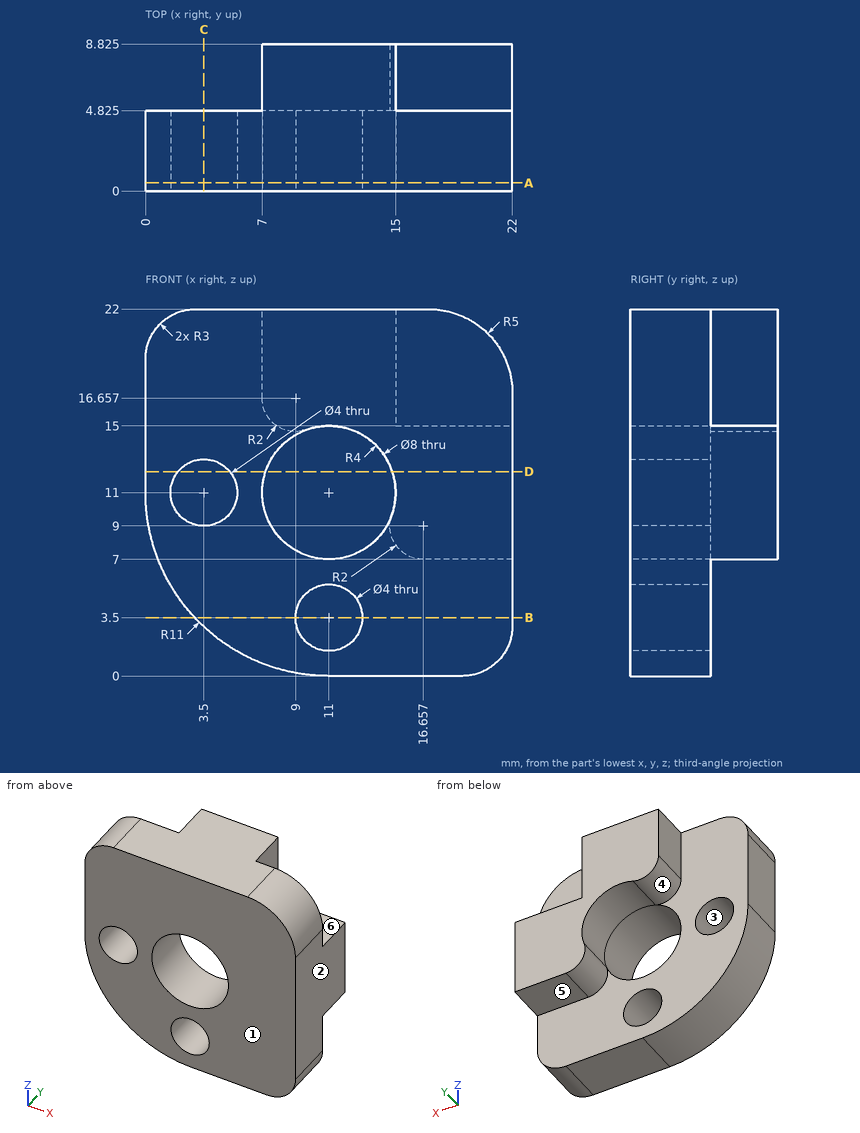
Geometry: see drawing. Coordinates: mm, zero at the bounding-box minimum. A direction names the side the tool comes from. Give positions to 0.01 mm unless a question says otherwise; leave off trailing zeros. Loops run counter-clockwise (first coordinate to the right, second up) from the corner with the lowest first, then second, coordinate; pieces in that order, holes last. Notation, with made-up numbers: M 22,27.5 L 29,27.5 A28 cw 29,61.5 Z; hole C -36.5,37 d8. An arc over 180 degrees is marked long. Use one line per item in the form item = value.
1. Pull-direction query (X, two-part tool) for the marked faces 1, 2 and 3; classes: released by +X, released by -X, zero draft, split by the parting line, or undercut.
Numbers:
face_1 = zero draft
face_2 = released by +X
face_3 = undercut
2. Section query B-B, the plane z = 3.5. Return the cut outline in (x, y) (1 decimal).
Numbers:
outline = M 3,0 L 9,0 L 9,4.8 L 3,4.8 Z; M 13,0 L 22,0 L 22,4.8 L 13,4.8 Z
3. Line query: L1, parallel to X at y = 1.3, z = 11; L2, parallel to Y at x = 4.25, z = 5.5 (3 decimals); L3, parallel to Z at x = 20, y = 7.5. Output: solid intervals per line, ascending.
Numbers:
L1 = 0 to 1.5, 5.5 to 7, 15 to 22
L2 = 0 to 4.825
L3 = 7 to 15
4. Section query D-D, the plane z = 12.25. Return the cut outline in (x, y) (1 decimal), and give its area (3 significant figures).
Numbers:
outline = M 0,0 L 1.9,0 L 1.9,4.8 L 0,4.8 Z; M 5.1,0 L 7.2,0 L 7.2,4.8 L 5.1,4.8 Z; M 14.8,0 L 22,0 L 22,8.8 L 14.8,8.8 Z
area = 83.2 mm²
5. First-contact query: pin 1 (1.5 mm diameter, centred on y = 6, z = 3.5, fed in from -X); pin 2 (4.5 mm diameter, centred on x = 18, y = 7.5, fed in from +Z); pin 3 (3 mm diameter, centred on y = 7.5, z = 18.5, fed in from +X); pin 4 (6 mm diameter, centred on x = 11, z = 3, fed in from +Y) (3 decimals). Flat tips, straight axial feed; report the tip coordinate or a pass-through.
Numbers:
pin_1 = through
pin_2 = 15
pin_3 = 15
pin_4 = 4.825
6. Section query C-C, the plane x = 3.5. Return the cut outline in (y, z) (1 decimal), and give its area (3 significant figures).
Numbers:
outline = M 0,3 L 4.8,3 L 4.8,9 L 0,9 Z; M 0,13 L 4.8,13 L 4.8,22 L 0,22 Z
area = 72.6 mm²
7. Reachability of the marked faces 4, 5 and 6 from +Z, -Z, +X, -X, +Y, -Y: full face, straight path, thin tool, end or side. Return the list, or none.
Numbers:
face_4 = -Z, +Y
face_5 = -Z, +X, -X, +Y
face_6 = +Z, +X, +Y
8. Section query A-A, the plane y = 0.5. Return the cut outline in (x, z), and give its area (3 significant figures).
Numbers:
outline = M 0,11 A11 ccw 11,0 L 19,0 A3 ccw 22,3 L 22,17 A5 ccw 17,22 L 3,22 A3 ccw 0,19 Z; hole C 3.5,11 d4; hole C 11,11 d8; hole C 11,3.5 d4
area = 373 mm²
